Input: part model. Units: mm. Frame: model coordinates. A direction names the side the tool comes from. Round coordinates to 2 decimals unless told otherwise and drop trailing zeros. Loops run counter-clockwise (first coordinate to the right, second up) from the corner with the lowest first, then second, coordinate; pieces in that order, holes last. Notation, with made-up numbers: (19.5, 67) -> (70.5, 67) arc R17 cw to (70.5, 73) -> close; hole circle Ø10 at (21.5, 37.5). An arc over 180 degrees is marked (long way). Answer as a JSON object with one key per item and string values. Group by question number.
Item 1: Section query A-A on z = 2.5. Return loops of the section in (x, y), and give its area (3 significant figures).
Item 2: Set-up query: faces 4 (the cylindrical face through (32.049, 5.141, -22.096)), 5 (the flat face through (11.86, 20.82, -0.5)). Return all of +Z, -Z, +X, -X, +Y, -Y with unobstructed straight access to the full face (end or side cutting, diameter ignored); none if empty.
Item 3: Pin query (flat end, axial travel): pin 1 (2 mm diameter, centred on y = 30, z = -5, fed in from -X); pin 2 (1 mm diameter, centred on y = 25.5, z = 9.5, fed in from -X); pin 3 (4 mm diameter, centred on x = 26.5, z = -19.5, fed in from +Y). Return the tip coordinate at first contact, or that it passes through.
Item 4: Section query B-B on z = -24. Return loops of the section in (x, y), and give its area (3 significant figures).
Item 5: Section query C-C on y = 13. Count the separate pieces of the cut face and the enclosed holes in it, and give its area (3 significant figures).
Item 6: Material intervals for line 1 (Z direction, x = 9, y = 24.5); line 2 (X direction, y = 12, z = 25); line 3 (Z direction, x = 39, y = 20), sorted ascending. Write a range as [from, to].
Item 7: Draft query along X for faces 1 (the cylindrical face through (5.02, 12.15, 5.08)), 2 (the flat face through (35, 16, 34.5)), 3 (the flat face through (41.895, 19.913, -1.497)). Return one class per face: released by +X, released by -X, zero draft, split by the parting line, or undercut.
from build123d import *

# Parameters (mm, degrees)
SKETCH1_W           = 71
SKETCH1_H           = 38
SKETCH1_R           = 12
SKETCH1_R_2         = 8
BOSS_EXTRUDE1_DEPTH = 40
SKETCH7_R           = 16
CUT_EXTRUDE4_DEPTH  = 7
SKETCH8_R           = 14
CUT_EXTRUDE5_DEPTH  = 8
CUT_EXTRUDE6_START  = -7
SKETCH9_R           = 16
CUT_EXTRUDE6_DEPTH  = 7
CUT_EXTRUDE7_START  = -8
SKETCH10_R          = 14
CUT_EXTRUDE7_DEPTH  = 8
CUT_EXTRUDE8_DEPTH  = 92.306031742


with BuildPart() as part:
    # Sketch1 → Boss-Extrude1 (new body)
    with BuildSketch(Plane(origin=(0, 0, 0), x_dir=(0, 0, 1), z_dir=(-0.9961946980917459, 0.08715574274765504, 0))):
        with Locations((-1, 19)):
            Rectangle(SKETCH1_W, SKETCH1_H)
        with Locations(Location((-17.5, 19, 0), (0, 0, 270))):
            Circle(SKETCH1_R, mode=Mode.SUBTRACT)
        with Locations(Location((17.5, 19, 0), (0, 0, 270))):
            Circle(SKETCH1_R_2, mode=Mode.SUBTRACT)
    extrude(amount=-BOSS_EXTRUDE1_DEPTH)

    # Sketch7 → Cut-Extrude4 (cut)
    with BuildSketch(Plane(origin=(0, 0, 0), x_dir=(0, 0, 1), z_dir=(-0.9961946980917459, 0.08715574274765503, 0))):
        with Locations(Location((-17.5, 19, 0), (0, 0, 270))):
            Circle(SKETCH7_R)
    extrude(amount=-CUT_EXTRUDE4_DEPTH, mode=Mode.SUBTRACT)

    # Sketch8 → Cut-Extrude5 (cut)
    with BuildSketch(Plane(origin=(0, 0, 0), x_dir=(0, 0, 1), z_dir=(-0.9961946980917459, 0.08715574274765503, 0))):
        with Locations(Location((17.5, 19, 0), (0, 0, 270))):
            Circle(SKETCH8_R)
    extrude(amount=-CUT_EXTRUDE5_DEPTH, mode=Mode.SUBTRACT)

    # Sketch9 → Cut-Extrude6 (cut)
    with BuildSketch(Plane(origin=(39.847787924, -3.48622971, 0), x_dir=(0, 0, -1), z_dir=(0.9961946980917459, -0.08715574274765503, 0)).offset(CUT_EXTRUDE6_START)):
        with Locations(Location((17.5, 19, 0), (0, 0, 270))):
            Circle(SKETCH9_R)
    extrude(amount=CUT_EXTRUDE6_DEPTH, mode=Mode.SUBTRACT)

    # Sketch10 → Cut-Extrude7 (cut)
    with BuildSketch(Plane(origin=(39.847787924, -3.48622971, 0), x_dir=(0, 0, -1), z_dir=(0.9961946980917459, -0.08715574274765503, 0)).offset(CUT_EXTRUDE7_START)):
        with Locations(Location((-17.5, 19, 0), (0, 0, 270))):
            Circle(SKETCH10_R)
    extrude(amount=CUT_EXTRUDE7_DEPTH, mode=Mode.SUBTRACT)

    # Sketch11 → Cut-Extrude8 (cut, through all)
    with BuildSketch(Plane.XY.offset(34.5)):
        Polygon((13.273865205, 36.9838411), (33.197759167, 35.240726245), (30.408775399, 3.362495906), (10.484881437, 5.105610761), align=None)
    extrude(amount=-CUT_EXTRUDE8_DEPTH, mode=Mode.SUBTRACT)


solid = part.part
Solved:
{
 "1": {"outline": "(0, 0) -> (39.85, -3.49) -> (43.16, 34.37) -> (33.2, 35.24) -> (30.41, 3.36) -> (10.48, 5.11) -> (13.27, 36.98) -> (3.31, 37.86) -> close", "area": "880 mm²"},
 "2": {"face 4": "none", "face 5": "+Z, -Z"},
 "3": {"pin 1": "x = 2.54", "pin 2": "x = 10.22", "pin 3": "y = 3.88"},
 "4": {"outline": "(0, 0) -> (39.85, -3.49) -> (40.23, 0.88) -> (33.26, 1.49) -> (33.65, 6) -> (30.66, 6.26) -> (30.41, 3.36) -> (10.48, 5.11) -> (10.74, 8.01) -> (7.75, 8.27) -> (7.36, 3.75) -> (0.38, 4.36) -> close; (2.93, 33.49) -> (9.9, 32.88) -> (9.51, 28.37) -> (12.5, 28.1) -> (13.27, 36.98) -> (3.31, 37.86) -> close; (32.42, 26.36) -> (35.41, 26.1) -> (35.8, 30.62) -> (42.78, 30.01) -> (43.16, 34.37) -> (33.2, 35.24) -> close", "area": "350 mm²"},
 "5": {"separate pieces": "6", "enclosed holes": "0", "area": "379 mm²"},
 "6": {"line 1": "[-36.5, -32.25], [-2.75, 4.94], [30.06, 34.5]", "line 2": "[9.08, 11.09], [31.16, 33.17]", "line 3": "[-36.5, -32.9], [-2.1, 4.18], [30.82, 34.5]"},
 "7": {"face 1": "undercut", "face 2": "zero draft", "face 3": "released by +X"}
}
